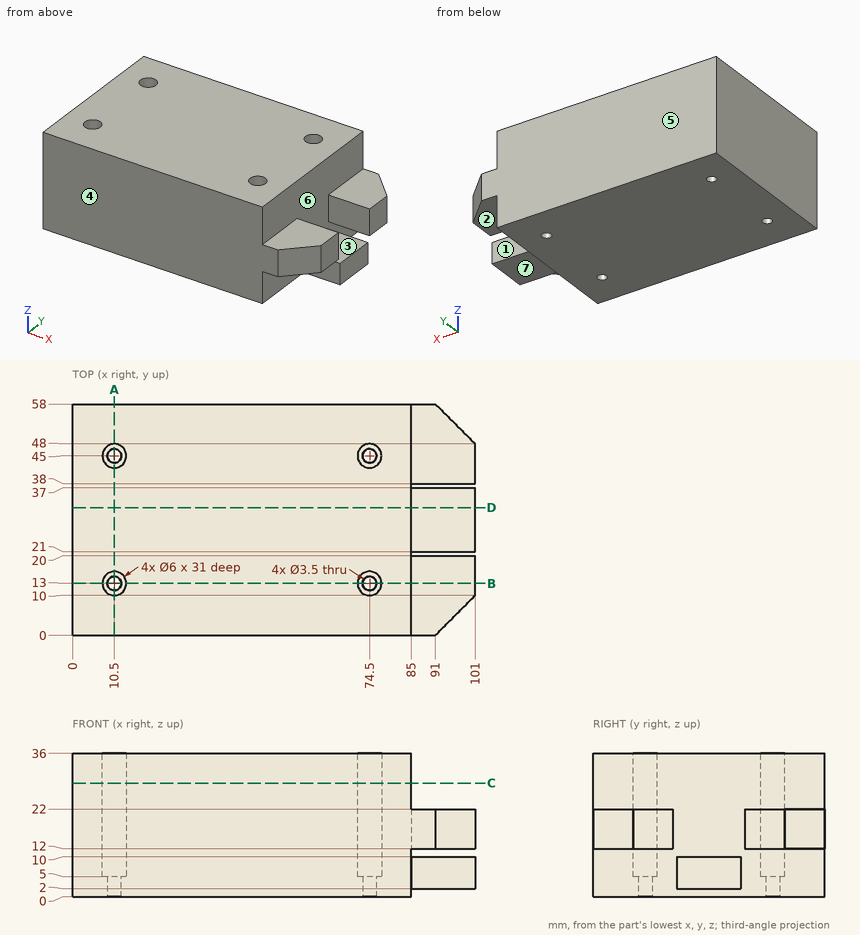
Design review of the part shown in the three views and the two pictorial views. Dimensions are in mm from the part's minimum x, y and z. A direction names the side the tool comes from. Coordinates: 2 decimals unless noted, no trailing zeros. Write each loop counter-clockwise with the first axis right and the second up, starting at its lowest first coordinate (ties: lowest second). Pieces come first, ordered by that corner, then holes.
1) To check wall thickness, follow probe 1 along Y at (x, z) = (10.5, 2); probe 2 along X at (y, z) = (13, 1.95); probe 3 along Y at (x, z) = (74.5, 21.5). State the ranges of each line that lie inside material, in increasing order.
2) We need section C-C on z = 28.5. State the section outline as (x, y) points, then the cut area to 3 significant figures.
3) We need section D-D on y = 32. State the section outline as (x, z) points, then the cut area to 3 significant figures.
4) We need section B-B on y = 13. State the section outline as (x, z) points.
5) Clearance check with flat-ended pins moving along their axes: pin 1 Ø8 at (x, y) = (92.5, 50) entering from -Z; pin 2 Ø5 at (x, y) = (74.5, 13) entering from +Z; pin 3 Ø5 at (x, y) = (91, 44) entering from +Z. State where each tip first meets the part, or that it passes through.
6) We need section A-A on x = 10.5. State the section outline as (y, z) points, then the cut area to 3 significant figures.
7) Machinability: for the marked faces 1, 2 and 3, which of the approach directions +Z, -Z, +X, -X, +Y, -Y give a long, thin tool a straight path to every point of the face, cutting with its end or side? Answer none if there is none.
8) The part is to be moulded in two halves that separate along Y. For the marked faces 4, 5, 6 and 7, say which applies: pulls with the +Y half, pulls with the -Y half, needs draft (parallel to the pull), parting line crosses it, or undercut.
Answer list:
1. probe 1: y = 0 to 11.25, 14.75 to 43.25, 46.75 to 58
1. probe 2: x = 0 to 8.75, 12.25 to 72.75, 76.25 to 85
1. probe 3: y = 0 to 10, 16 to 42, 48 to 58
2. outline: (0, 0) - (85, 0) - (85, 58) - (0, 58) - close; hole circle Ø6 at (10.5, 13); hole circle Ø6 at (10.5, 45); hole circle Ø6 at (74.5, 13); hole circle Ø6 at (74.5, 45)
2. area: 4,820 mm2
3. outline: (0, 0) - (85, 0) - (85, 2) - (101, 2) - (101, 10) - (85, 10) - (85, 36) - (0, 36) - close
3. area: 3,190 mm2
4. outline: (0, 0) - (8.75, 0) - (8.75, 5) - (7.5, 5) - (7.5, 36) - (0, 36) - close; (12.25, 0) - (72.75, 0) - (72.75, 5) - (71.5, 5) - (71.5, 36) - (13.5, 36) - (13.5, 5) - (12.25, 5) - close; (76.25, 0) - (85, 0) - (85, 12) - (101, 12) - (101, 22) - (85, 22) - (85, 36) - (77.5, 36) - (77.5, 5) - (76.25, 5) - close
5. pin 1: stops at z = 12
5. pin 2: stops at z = 5
5. pin 3: stops at z = 22
6. outline: (0, 0) - (11.25, 0) - (11.25, 5) - (10, 5) - (10, 36) - (0, 36) - close; (14.75, 0) - (43.25, 0) - (43.25, 5) - (42, 5) - (42, 36) - (16, 36) - (16, 5) - (14.75, 5) - close; (46.75, 0) - (58, 0) - (58, 36) - (48, 36) - (48, 5) - (46.75, 5) - close
6. area: 1,680 mm2
7. face 1: +Z, -Z, +X, +Y
7. face 2: -Z, +X, +Y, -Y
7. face 3: +Z, +X, +Y, -Y
8. face 4: pulls with the -Y half
8. face 5: pulls with the +Y half
8. face 6: undercut
8. face 7: needs draft
